Work out the finished part from the listing and answer in its coordinate system (mm). A direction names the side the tool comes from. Give positions to 0.01 mm unless a question says otherwise; leave off trailing zeros. Write each loop counter-clockwise with the first axis right and the second up, starting at its lowest first coordinate (ties: lowest second). Pieces come first, ordered by that corner, then holes. Notation, with made-up numbers: (-24.5, 45) - (24.5, 45) arc R23 ccw to (24.5, 58) - close; hole circle Ø7 at (51, 11.5). An arc over 180 degrees is marked (long way). Write item = value, one per line.
from build123d import *

# Parameters (mm, degrees)
IZIM2_R                     = 27.5
Y_KSEKLIK_EKSTR_ZYON1_DEPTH = 5
Y_KSEKLIK_EKSTR_ZYON1_TAPER = 5
IZIM4_R                     = 3.625
KES_EKSTR_ZYON1_DEPTH       = 2.4
IZIM4_3_R                   = 2.35
KES_EKSTR_ZYON2_DEPTH       = 14
KES_EKSTR_ZYON3_DEPTH       = 3.2
KES_EKSTR_ZYON4_DEPTH       = 3.5
SKETCH1_R                   = 4
BOSS_EXTRUDE1_DEPTH         = 5
SKETCH3_R                   = 2.2
CUT_EXTRUDE1_DEPTH          = 5.2
CHAMFER1_SIZE               = 2.5


with BuildPart() as part:
    # izim2 → Y_kseklik-Ekstr_zyon1 (new body)
    with BuildSketch(Plane(origin=(0, 0, 0), x_dir=(1, 0, 0), z_dir=(0, 1, 0))):
        Circle(IZIM2_R)
    extrude(amount=Y_KSEKLIK_EKSTR_ZYON1_DEPTH, taper=Y_KSEKLIK_EKSTR_ZYON1_TAPER)

    # izim4 → Kes-Ekstr_zyon1 (cut)
    with BuildSketch(Plane.XZ):
        with BuildLine():
            Line((2.2, -3.691961397), (15.927868459, -2.388197354))
            ThreePointArc((15.927868459, -2.388197354), (18.1, 0), (15.927868459, 2.388197354))
            Line((15.927868459, 2.388197354), (2.2, 3.691961397))
            Line((2.2, 3.691961397), (2.2, 7.45))
            ThreePointArc((2.2, 7.45), (0, 9.65), (-2.2, 7.45))
            Line((-2.2, 7.45), (-2.2, 3.691961397))
            Line((-2.2, 3.691961397), (-15.927868459, 2.388197354))
            ThreePointArc((-15.927868459, 2.388197354), (-18.1, 0), (-15.927868459, -2.388197354))
            Line((-15.927868459, -2.388197354), (-2.2, -3.691961397))
            Line((-2.2, -3.691961397), (-2.2, -7.45))
            ThreePointArc((-2.2, -7.45), (0, -9.65), (2.2, -7.45))
            Line((2.2, -7.45), (2.2, -3.691961397))
        make_face()
        with Locations(Location((0, 0, 0), (0, 0, 270))):
            Circle(IZIM4_R, mode=Mode.SUBTRACT)
    extrude(amount=-KES_EKSTR_ZYON1_DEPTH, mode=Mode.SUBTRACT)

    # izim4_3 → Kes-Ekstr_zyon2 (cut)
    with BuildSketch(Plane.XZ):
        with Locations(Location((0, 0, 0), (0, 0, 270))):
            Circle(IZIM4_3_R)
    extrude(amount=-KES_EKSTR_ZYON2_DEPTH, mode=Mode.SUBTRACT)

    # izim8 → Kes-Ekstr_zyon3 (cut)
    with BuildSketch(Plane.XZ):
        Polygon((-5, 3.426039609), (-5, -3.426039609), (-2.2, -3.691961397), (2.2, -3.691961397), (5, -3.426039609), (5, 3.426039609), (2.2, 3.691961397), (-2.2, 3.691961397), align=None)
    extrude(amount=-KES_EKSTR_ZYON3_DEPTH, mode=Mode.SUBTRACT)

    # izim9 → Kes-Ekstr_zyon4 (cut)
    with BuildSketch(Plane.XZ.offset(-2.4)):
        with BuildLine():
            Line((12.262809511, -0.8), (8.262809511, -0.8))
            ThreePointArc((8.262809511, -0.8), (7.462809511, 0), (8.262809511, 0.8))
            Line((8.262809511, 0.8), (12.262809511, 0.8))
            ThreePointArc((12.262809511, 0.8), (13.062809511, 0), (12.262809511, -0.8))
        make_face()
        with BuildLine():
            Line((-12.262809511, -0.8), (-8.262809511, -0.8))
            ThreePointArc((-8.262809511, -0.8), (-7.462809511, 0), (-8.262809511, 0.8))
            Line((-8.262809511, 0.8), (-12.262809511, 0.8))
            ThreePointArc((-12.262809511, 0.8), (-13.062809511, 0), (-12.262809511, -0.8))
        make_face()
    extrude(amount=-KES_EKSTR_ZYON4_DEPTH, mode=Mode.SUBTRACT)

    # Sketch1 → Boss-Extrude1 (add)
    with BuildSketch(Plane.XZ):
        with Locations(Location((-13, 10.5, 0), (0, 0, 90))):
            Circle(SKETCH1_R)
        with Locations(Location((13, 10.5, 0), (0, 0, 90))):
            Circle(SKETCH1_R)
        with Locations(Location((13, -10.5, 0), (0, 0, 90))):
            Circle(SKETCH1_R)
        with Locations(Location((-13, -10.5, 0), (0, 0, 90))):
            Circle(SKETCH1_R)
    extrude(amount=BOSS_EXTRUDE1_DEPTH)

    # Sketch3 → Cut-Extrude1 (cut)
    with BuildSketch(Plane(origin=(0, 5, 0), x_dir=(1, 0, 0), z_dir=(0, 1, 0))):
        with Locations(Location((13, 10.5, 0), (0, 0, 270))):
            Circle(SKETCH3_R)
        with Locations(Location((-13, 10.5, 0), (0, 0, 270))):
            Circle(SKETCH3_R)
        with Locations(Location((-13, -10.5, 0), (0, 0, 270))):
            Circle(SKETCH3_R)
        with Locations(Location((13, -10.5, 0), (0, 0, 270))):
            Circle(SKETCH3_R)
    extrude(amount=-CUT_EXTRUDE1_DEPTH, mode=Mode.SUBTRACT)

    # Chamfer1
    chamfer1_edges = [part.edges().sort_by_distance(p)[0] for p in [
        (-13, 0, 6.5),
        (13, 0, 6.5),
        (13, 0, -14.5),
        (-13, 0, -14.5),
    ]]
    chamfer(chamfer1_edges, length=CHAMFER1_SIZE)


solid = part.part
1. Given pin 1 (3 mm diameter, centred on x = 16, z = 17.5, fed in from -Y); pin 2 (1 mm diameter, centred on x = 0.5, y = 2.5, fed in from +Z); pin 3 (0.7 mm diameter, centred on y = 0.5, z = 5, fed in from -X), each flat-ended and moving along its own axis, determine where each tip first touches the part or whether it passes through.
Solution:
pin_1 = -0.38
pin_2 = 27.32
pin_3 = -27.07
2. Find section A-A, the plane x = 0. Give the vertices of the cut face in (y, z).
Solution:
outline = (0, -27.5) - (5, -27.06) - (5, -2.35) - (3.2, -2.35) - (3.2, -3.69) - (2.4, -3.69) - (2.4, -9.65) - (0, -9.65) - close; (0, 9.65) - (2.4, 9.65) - (2.4, 3.69) - (3.2, 3.69) - (3.2, 2.35) - (5, 2.35) - (5, 27.06) - (0, 27.5) - close
3. A tool of negligible diameter and unlimited length cuts with its end or side. For faces 1 (the cylindrical face through (-18.1, 1.2, 0)), 2 (the cylindrical face through (14.855, 2.436, 11.683)), 3 (the flat face through (6, 5, 0)), 4 (the flat face through (-10, 4, -0.8)), from which of +Z, -Z, +X, -X, +Y, -Y can it reach the whole face along a straight path? Write none if from no direction.
Solution:
face_1 = -Y
face_2 = +Y
face_3 = +Z, -Z, +X, -X, +Y
face_4 = +Y, -Y
4. Straight lines are drawn through the part: line 1 (X direction, y = 3.3, z = -10.5); line 2 (X direction, y = 3.9, z = -10.5); line 3 (Z direction, x = 15, y = 4.75). For each, find the intervals that lie inside material, in ascending order.
Solution:
line_1 = -25.1 to -15.2, -10.8 to 10.8, 15.2 to 25.1
line_2 = -25.05 to -15.2, -10.8 to 10.8, 15.2 to 25.05
line_3 = -22.55 to -11.42, -9.58 to 9.58, 11.42 to 22.55
5. For a pull along X with two mould halves and no side action, classify faces 5 (the flat face through (13, -5, -11)), 6 (the cylindrical face through (0.71, 4.09, -2.24)), 7 (the conical face through (-5.87, 4.76, 26.44)), 8 (the conical face through (-14.24, -2.38, -6.57)) as pulls with the +X half, pulls with the -X half, needs draft (parallel to the pull), parting line crosses it, or undercut.
Solution:
face_5 = needs draft
face_6 = undercut
face_7 = parting line crosses it
face_8 = undercut
